CAD build for the part. Positions are in the model's coordinates, mm. Round coordinates to 2 decimals unless told otherwise and drop trailing zeros. Write each loop counter-clockwise with the first axis right and the second up, starting at its lowest first coordinate (ties: lowest second). Pieces come first, ordered by that corner, then holes. Notation, with made-up numbers: (21, 88.5) -> (37, 88.5) arc R24 cw to (37, 111.5) -> close; hole circle Ø10 at (9.5, 48). An arc over 180 degrees is marked (long way). Put each result on its own line as item: value. Start each with the question number.
1. Saw through at C-C on z = -298. List the corners of the cut face in (x, y).
2. Saw through at A-A on y = 1.05. List the corners of the cut face in (x, z).
3. Flat gauge pin, fed straight in: P1, Ø0.6, axis at x = -59.5, y = 1, coming from the -Z side. Where does the tip first touch, or does it go through?
4. Saw through at B-B on x = -59.5. List the corners of the cut face in (y, z), and give its area (3 significant figures).
5. Drill centre lines: line 1 (X direction, y = 1.15, z = -174); line 2 (Z direction, x = -58.5, y = 1.7). Where is each one in solid material? Low to high. Write a range as from..to.
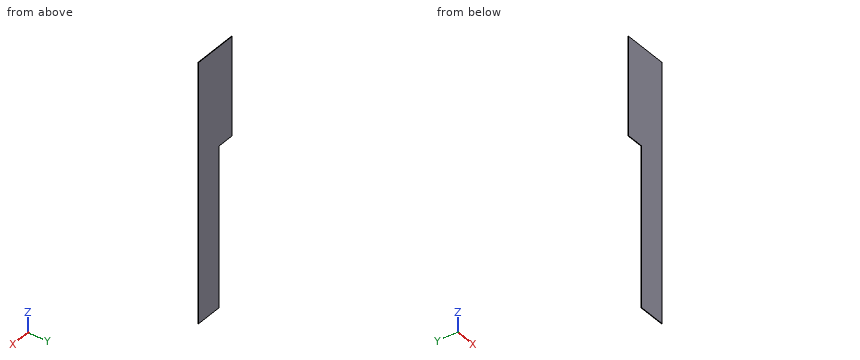
Autodesk Inventor part; units mm, degrees
ref_plane "YZ Plane" through (0, 0, 0) normal (1, 0, 0) x (0, 1, 0)
ref_plane "XZ Plane" through (0, 0, 0) normal (0, 1, 0) x (-1, 0, 0)
ref_plane "XY Plane" through (0, 0, 0) normal (0, 0, 1) x (1, 0, 0)
sketch "Sketch1" plane through (0, 0, 0) normal (0, 1, 0) x (-1, 0, 0)
  line L0 (20, -525) -> (-90, -525)
  line L1 (-90, 525) -> (90, 525)
  line L2 (0, 525) -> (0, -525)
  line L3 (20, -525) -> (20, 125)
  line L4 (20, 125) -> (90, 125)
  line L5 (90, 525) -> (90, 125)
  line L6 (20, 0) -> (-90, 0)
  line L7 (-90, 525) -> (-90, -525)
  point P0 (0, 0)
  dimension "d6" = 1050
  dimension "d7" = 180
  dimension "d8" = 70
  dimension "d10" = 650
extrude "Extrusion1" add sketch "Sketch1" along normal blind 2
properties part number "Mi" material "LCP Plastic"
Return value:
1. outline: (-20, 0) -> (90, 0) -> (90, 2) -> (-20, 2) -> close
2. outline: (-90, 125) -> (-20, 125) -> (-20, -525) -> (90, -525) -> (90, 525) -> (-90, 525) -> close
3. P1: stops at z = 125
4. outline: (0, 125) -> (2, 125) -> (2, 525) -> (0, 525) -> close
4. area: 800 mm^2
5. line 1: x = -20..90
5. line 2: z = 125..525
